```python
from build123d import *

# Parameters (mm, degrees)
SKETCH2_W               = 14
SKETCH2_H               = 8
CUT_EXTRUDE1_DEPTH      = 6.5
CUT_EXTRUDE1_DEPTH_BACK = 6.5
CHAMFER1_SIZE           = 0.25


with BuildPart() as part:
    # Sketch1 → Revolve1 (revolve)
    with BuildSketch(Plane.XY):
        Polygon((3.925, 1.6256), (3.925, 12.4), (2.4, 12.4), (2.4, 0.2), (2.6, 0), (5.5, 0), (5.5, 1.6256), align=None)
    revolve(axis=Axis((0, 0, 0), (0, -1, 0)))

    # Sketch2 → Cut-Extrude1 (cut, two sides)
    with BuildSketch(Plane.XY) as cut_extrude1_sk:
        with Locations((0, 9)):
            Rectangle(SKETCH2_W, SKETCH2_H)
    extrude(amount=CUT_EXTRUDE1_DEPTH, mode=Mode.SUBTRACT)
    extrude(cut_extrude1_sk.sketch, amount=-CUT_EXTRUDE1_DEPTH_BACK, mode=Mode.SUBTRACT)

    # Chamfer1
    chamfer1_edges = [part.edges().sort_by_distance(p)[0] for p in [
        (-3.925, 5, 0),
        (-2.4, 5, 0),
    ]]
    chamfer(chamfer1_edges, length=CHAMFER1_SIZE)


solid = part.part
```
The model under review builds one solid part; all positions refer to its coordinate system, in mm. A direction names the side the tool comes from. Round coordinates to 2 decimals unless told otherwise and drop trailing zeros. Loops run counter-clockwise (first coordinate to the right, second up) from the corner with the lowest first, then second, coordinate; pieces in that order, holes last.
Item 1: For faces 1 (the face through (-2.893, 3.21, 2.653)), 2 (the face through (3, 0, -1)), list the 3-axis set-ups (+Z, -Z, +X, -X, +Y, -Y) from which the entire face can be reached by the end or side of a thin tool; tool diameter is ignored.
Determined:
face 1: +Y
face 2: +Z, -Z, +X, -X, -Y
Item 2: Take a section at D-D (y = 3.25). Write out the cut boundary in (x, z) (3 decimals).
Determined:
outline: circle Ø7.85 at (0, 0); hole circle Ø4.8 at (0, 0)
Item 3: Take a section at A-A (x = 0). Write out the cut boundary in (y, z) (3 decimals).
Determined:
outline: (0, -5.5) - (1.626, -5.5) - (1.626, -3.925) - (4.75, -3.925) - (5, -3.675) - (5, -2.65) - (4.75, -2.4) - (0.2, -2.4) - (0, -2.6) - close; (0, 2.6) - (0.2, 2.4) - (4.75, 2.4) - (5, 2.65) - (5, 3.675) - (4.75, 3.925) - (1.626, 3.925) - (1.626, 5.5) - (0, 5.5) - close
Item 4: For line 1 (Z direction, x = 0, y = 2.5) (3 decimals); line 2 (Z direction, x = 0, y = 1.3); line 3 (Y direction, x = 2, z = -3.75), list the stretches that pass through material, from the lowest coordinate up.
Determined:
line 1: z = -3.925 to -2.4, 2.4 to 3.925
line 2: z = -5.5 to -2.4, 2.4 to 5.5
line 3: y = 0 to 1.63
Item 5: Clearance check with flat-ended pins moving along their axes: pin 1 Ø1 at (y, z) = (1, -1.5) entering from -X; pin 2 Ø2 at (y, z) = (3, 3) entering from -X; pin 3 Ø1 at (x, y) = (-3, 2.5) entering from +Z. State where each tip first meets the part, or that it passes through.
Determined:
pin 1: stops at x = -5.41
pin 2: stops at x = -3.38
pin 3: stops at z = 3.03
Item 6: Take a section at B-B (z = 0). Write out the cut boundary in (x, y) (3 decimals).
Determined:
outline: (-5.5, 0) - (-2.6, 0) - (-2.4, 0.2) - (-2.4, 4.75) - (-2.65, 5) - (-3.675, 5) - (-3.925, 4.75) - (-3.925, 1.626) - (-5.5, 1.626) - close; (2.4, 0.2) - (2.6, 0) - (5.5, 0) - (5.5, 1.626) - (3.925, 1.626) - (3.925, 4.75) - (3.675, 5) - (2.65, 5) - (2.4, 4.75) - close
Item 7: Take a section at C-C (y = 1.4). Write out the cut boundary in (x, z), then the cut area to 3 significant figures.
Determined:
outline: circle Ø11 at (0, 0); hole circle Ø4.8 at (0, 0)
area: 76.9 mm2
Item 8: Mouldability with a two-part tool opening along X and no side actions: class faces 3 (the face through (2, 5, -2)), 4 (the face through (1.29, 2.443, 2.024)), 5 (the face through (-1.19, 0.82, -5.37)) as released by +X, released by -X, zero draft, split by the parting line, or undercut.
Determined:
face 3: zero draft
face 4: undercut
face 5: split by the parting line
